from build123d import *

# Parameters (mm, degrees)
SKETCH1_R           = 25.000000000000004
SKETCH1_R_2         = 1.9999999999993712
SKETCH1_R_3         = 2.0000000000000036
SKETCH1_R_4         = 2.0000000000002736
SKETCH1_R_5         = 1.9999999999996778
BOSS_EXTRUDE1_DEPTH = 4
SKETCH2_R           = 25
SKETCH2_R_2         = 22.50000000000001
BOSS_EXTRUDE2_DEPTH = 15
BOSS_EXTRUDE7_REACH = 78.843
SKETCH4_W           = 49.955357531530346
SKETCH4_H           = 19
BOSS_EXTRUDE8_DEPTH = 40
SKETCH7_R           = 2.499999999999995
SKETCH7_R_2         = 2.5000000000000004
CUT_EXTRUDE1_DEPTH  = 123.01861707374391
FILLET1_R           = 5
FILLET2_R           = 5


with BuildPart() as part:
    # Sketch1 → Boss-Extrude1 (new body)
    with BuildSketch(Plane(origin=(0, 0, 0), x_dir=(1, 0, 0), z_dir=(0, 1, 0))):
        with Locations(Location((21.22072875619714, -40.09390888269783, 0), (0, 0, 270))):
            Circle(SKETCH1_R)
        with Locations(Location((29.646509797315062, -55.43197309716617, 0), (0, 0, 270))):
            Circle(SKETCH1_R_2, mode=Mode.SUBTRACT)
        with Locations(Location((36.558792970665294, -31.668127841580553, 0), (0, 0, 270))):
            Circle(SKETCH1_R_3, mode=Mode.SUBTRACT)
        with Locations(Location((12.794947715079665, -24.75584466823032, 0), (0, 0, 270))):
            Circle(SKETCH1_R_4, mode=Mode.SUBTRACT)
        with Locations(Location((5.8826645417294365, -48.51968992381595, 0), (0, 0, 270))):
            Circle(SKETCH1_R_5, mode=Mode.SUBTRACT)
        with BuildLine():
            ThreePointArc((8.810101512256844, -41.5859984952772), (17.729498538084204, -52.096463259335145), (30.894801565269475, -48.009862096604984))
            Line((30.894801565269475, -48.009862096604984), (33.63135600013741, -38.60181927011846))
            ThreePointArc((33.63135600013741, -38.60181927011846), (24.711958974310075, -28.091354506060547), (11.5466559471248, -32.177955668790645))
            Line((11.5466559471248, -32.177955668790645), (8.810101512256844, -41.5859984952772))
        make_face(mode=Mode.SUBTRACT)
    extrude(amount=BOSS_EXTRUDE1_DEPTH)

    # Sketch2 → Boss-Extrude2 (add)
    with BuildSketch(Plane.XZ):
        with Locations(Location((21.22070938805554, 40.093908619998004, 0), (0, 0, 270.77710591))):
            Circle(SKETCH2_R)
        with Locations(Location((21.22070938805554, 40.093908619998004, 0), (0, 0, 270))):
            Circle(SKETCH2_R_2, mode=Mode.SUBTRACT)
    extrude(amount=BOSS_EXTRUDE2_DEPTH)

    # Sketch4 → Boss-Extrude7 (add, up to next)
    with BuildSketch(Plane(origin=(-2.11468835096776, 0, 7.270119796296657), x_dir=(-0.9602043501309836, 0, -0.2792984174490354), z_dir=(0.2792984174490354, 0, -0.9602043501309836)), mode=Mode.PRIVATE) as boss_extrude7_sk1:
        with Locations((-31.573501878114026, -5.500000000000001)):
            Rectangle(SKETCH4_W, SKETCH4_H)
    boss_extrude7_tool1 = extrude(boss_extrude7_sk1.sketch, amount=-BOSS_EXTRUDE7_REACH, mode=Mode.PRIVATE) - part.part
    add(boss_extrude7_tool1.solids().sort_by_distance((28.202326, -5.5, 16.088549))[0])

    # Sketch5 → Boss-Extrude8 (add)
    with BuildSketch(Plane(origin=(-2.114688350967763, 0, 7.270119796296668), x_dir=(-0.9602043501309836, 0, -0.27929841744903544), z_dir=(0.27929841744903544, 0, -0.9602043501309836))):
        Polygon((13.404176887651147, 4), (-76.55118064387919, 4), (-76.55118064387919, -15), (13.404176887651147, -15), (13.404176887651147, -5.5), align=None)
    extrude(amount=BOSS_EXTRUDE8_DEPTH)

    # Sketch7 → Cut-Extrude1 (cut, through all)
    with BuildSketch(Plane(origin=(9.057248346993656, 1.8e-15, -31.13805420894269), x_dir=(-0.9602043501309836, 0, -0.27929841744903544), z_dir=(0.27929841744903544, 0, -0.9602043501309836))):
        with Locations((-66.55118064387919, -5.499999999999998)):
            Circle(SKETCH7_R)
        with Locations((3.4041768876511456, -5.499999999999997)):
            Circle(SKETCH7_R_2)
    extrude(amount=-CUT_EXTRUDE1_DEPTH, mode=Mode.SUBTRACT)

    # Fillet1
    fillet1_edges = [part.edges().sort_by_distance(p)[0] for p in [
        (76.9760566599285, -15, 9.446656401367687),
    ]]
    fillet(fillet1_edges, radius=FILLET1_R)

    # Fillet2
    fillet2_edges = [part.edges().sort_by_distance(p)[0] for p in [
        (-9.399468959434873, -15, -15.677732598250907),
        (-9.399468959434873, 4, -15.677732598250907),
        (76.9760566599285, 4, 9.446656401367687),
    ]]
    fillet(fillet2_edges, radius=FILLET2_R)


solid = part.part
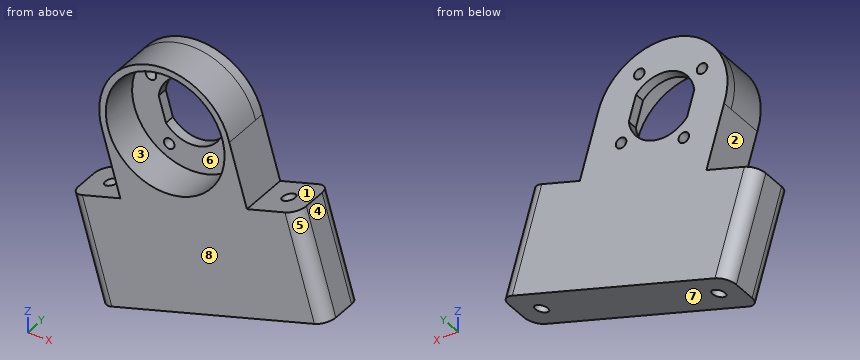
Verification items for the finished model (mm, model axes). Face numbers are marked on the shaded views. A direction names the side the tool comes from. Give positions to 0.01 mm unless a question says otherwise; leave off trailing zeros. Loops run counter-clockwise (first coordinate to the right, second up) from the corner with the lowest first, then second, coordinate; pieces in that order, holes last.
1) Depth check by flat-ended pin: pin 1 Ø2 at (y, z) = (-5, 7.5) entering from -X; pin 2 Ø6 at (x, y) = (0, -1) entering from +Z; pin 3 Ø1.5 at (y, z) = (-12, 20.5) entering from +X. Enter the tip coordinate at first touch or a pass-through.
2) Draft check along X on the marked faces 6, 7 and 8. Enter one of: pulls with the +X half, pulls with the -X half, needs draft (parallel to the pull), parting line crosses it, or undercut.
3) Set-up check for the marked faces 1, 2, 3, 4 and 5: record each of +Z, -Z, +X, -X, +Y, -Y from which the full face is reachable in a straight line by a thin tool's end or side.
4) Sectioned sample at C-C, the plane x = 50. Enter the section's corners in (y, z).
5) Thickness scan on line 1 along X through (y, z) = (-7, -6); line 2 along X through (y, z) = (-5, 26); line 3 along Z through (x, y) = (29, -8.5). Record the ranges inside material, lowest first.
Answers:
1. pin 1: stops at x = -3.34
1. pin 2: stops at z = 57.21
1. pin 3: stops at x = 73.69
2. face 6: undercut
2. face 7: pulls with the +X half
2. face 8: needs draft
3. face 1: +Z, +Y, -Y
3. face 2: -X, +Y, -Y
3. face 3: -Y
3. face 4: +Z, +X, +Y, -Y
3. face 5: +Z, +X, -Y
4. outline: (-15, -19.23) - (4, -19.23) - (4, 30.58) - (-15, 30.58) - close
5. line 1: x = -12.21 to -3.88, 0.28 to 68.97, 73.14 to 81.47
5. line 2: x = -0.69 to 3.68, 38.76 to 51.33, 64.3 to 72.16
5. line 3: z = -25.34 to 18.98, 61.21 to 63.85
